Here's the drawing with two shaded views (mm, measured from the low corner). I have some questions. Give positions to 0.01 mm unless a question says otherwise; leave off trailing zeros. Write each loop counter-clockwise with the first axis right and the second up, starting at its lowest first coordinate (ties: lowest second). Pieces come first, ordered by that corner, then holes. Notation, with made-up numbers: (-17, -13.5) -> (18, -13.5) arc R22 cw to (18, 25.5) -> close; hole circle Ø8 at (47, 51). An arc over 180 degrees is marked (long way). One line per item, written item: value.
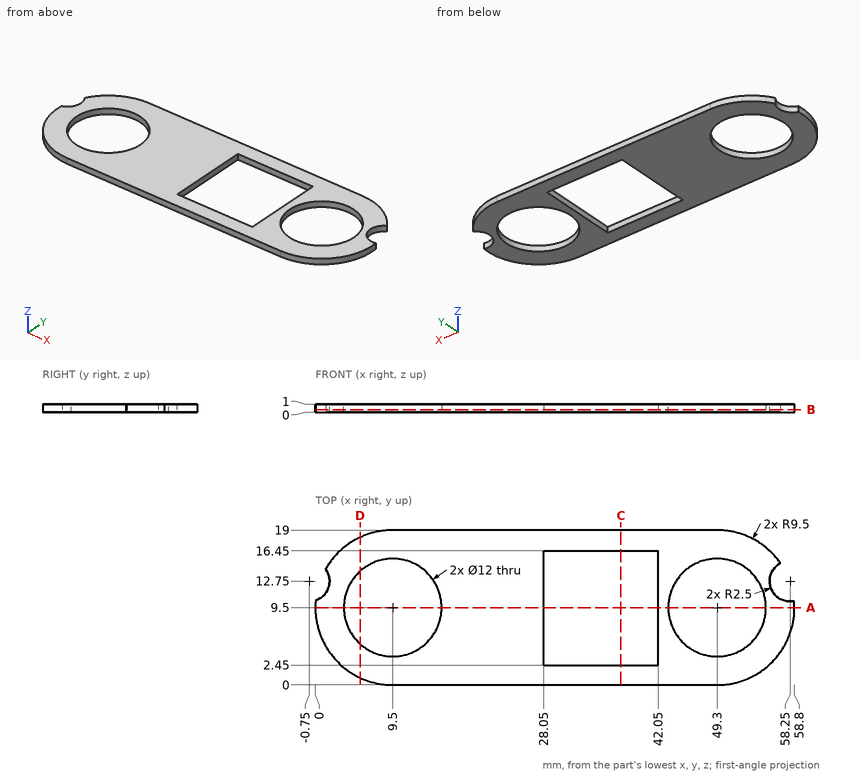
1) If we section it at B-B (z = 0.3): Write out the boundary of the cut face in (x, y), and give its area (3 significant figures).
Answer list:
outline: (0.04, 10.38) arc R9.5 ccw to (9.5, 0) -> (49.3, 0) arc R9.5 ccw to (58.77, 10.3) arc R2.5 cw to (57.08, 14.96) arc R9.5 ccw to (49.3, 19) -> (9.5, 19) arc R9.5 ccw to (1.26, 14.23) arc R2.5 cw to start; hole circle Ø12 at (9.5, 9.5); hole (28.05, 2.45) -> (42.05, 2.45) -> (42.05, 16.45) -> (28.05, 16.45) -> close; hole circle Ø12 at (49.3, 9.5)
area: 605 mm^2
2) If we section it at D-D (x = 5.5): Write out the boundary of the cut face in (y, z).
Answer list:
outline: (0.88, 0) -> (5.03, 0) -> (5.03, 1) -> (0.88, 1) -> close; (13.97, 0) -> (18.12, 0) -> (18.12, 1) -> (13.97, 1) -> close
3) I need wall thicknesses on L1, parallel to Y at x = 9.5, z = 0.5; L2, parallel to X at y = 4.75, z = 0.3; L3, parallel to X at y = 14.5, z = 0.2. Which ranges of each line are inside material? Lowest first, please.
Answer list:
L1: y = 0 to 3.5, 15.5 to 19
L2: x = 1.27 to 5.83, 13.17 to 28.05, 42.05 to 45.63, 52.97 to 57.53
L3: x = 1.42 to 6.18, 12.82 to 28.05, 42.05 to 45.98, 52.62 to 56.46
4) If we section it at C-C (x = 37.5): Write out the boundary of the cut face in (y, z).
Answer list:
outline: (0, 0) -> (2.45, 0) -> (2.45, 1) -> (0, 1) -> close; (16.45, 0) -> (19, 0) -> (19, 1) -> (16.45, 1) -> close
5) If we section it at A-A (y = 9.5): Write out the boundary of the cut face in (x, z), and give its area (3 significant figures).
Answer list:
outline: (0, 0) -> (3.5, 0) -> (3.5, 1) -> (0, 1) -> close; (15.5, 0) -> (28.05, 0) -> (28.05, 1) -> (15.5, 1) -> close; (42.05, 0) -> (43.3, 0) -> (43.3, 1) -> (42.05, 1) -> close; (55.3, 0) -> (58.8, 0) -> (58.8, 1) -> (55.3, 1) -> close
area: 20.8 mm^2
